Check sheet for the drawn part. Datum: minimum x, y, z corner. Units: mm. A direction names the side the tool comes from. Give positions to 0.01 mm unless a question says otherwise; leave off trailing zeros. Loops run counter-clockwise (first coordinate to the right, second up) from the corner with the lowest first, then second, coordinate; pieces in that order, holes last.
1. Cross-section at D-D, the plane x = 67.5. Record the cut outline in (y, z), plus the area to 3 significant figures.
2. Go/stop test with flat-tipped pins: pin 1 Ø5 at (y, z) = (22.5, 73.4) entering from -X; pin 2 Ø4 at (x, z) = (67.5, 12.5) entering from +Y; pin 3 Ø1.5 at (x, y) = (76.5, 78.5) entering from +Z; pin 4 Ø2.5 at (x, y) = (6.6, 22.5) entering from +Z. Record where each tip stops, or that it passes through.
3. Material ranges on L1, parallel to Z at x = 67.5, y = 14; L2, parallel to Y at x = 78.8, z = 12.5; L3, parallel to Y at x = 78, z = 12, recorded low to high.
4. Tool access check on the marked faces 1, 2 and 3. Record the directions out of +Z, -Z, +X, -X, +Y, -Y that give a thin tool (end or side, any length) a straight path to the whole face; none if there is none.
5. Cross-section at B-B, the plane x = 6.6. Record the cut outline in (y, z), plus the area to 3 significant figures.
6. Cross-section at A-A, the plane y = 22.5. Record the cut outline in (x, z).
7. Cross-section at C-C, the plane z = 73.4. Record the cut outline in (x, y).
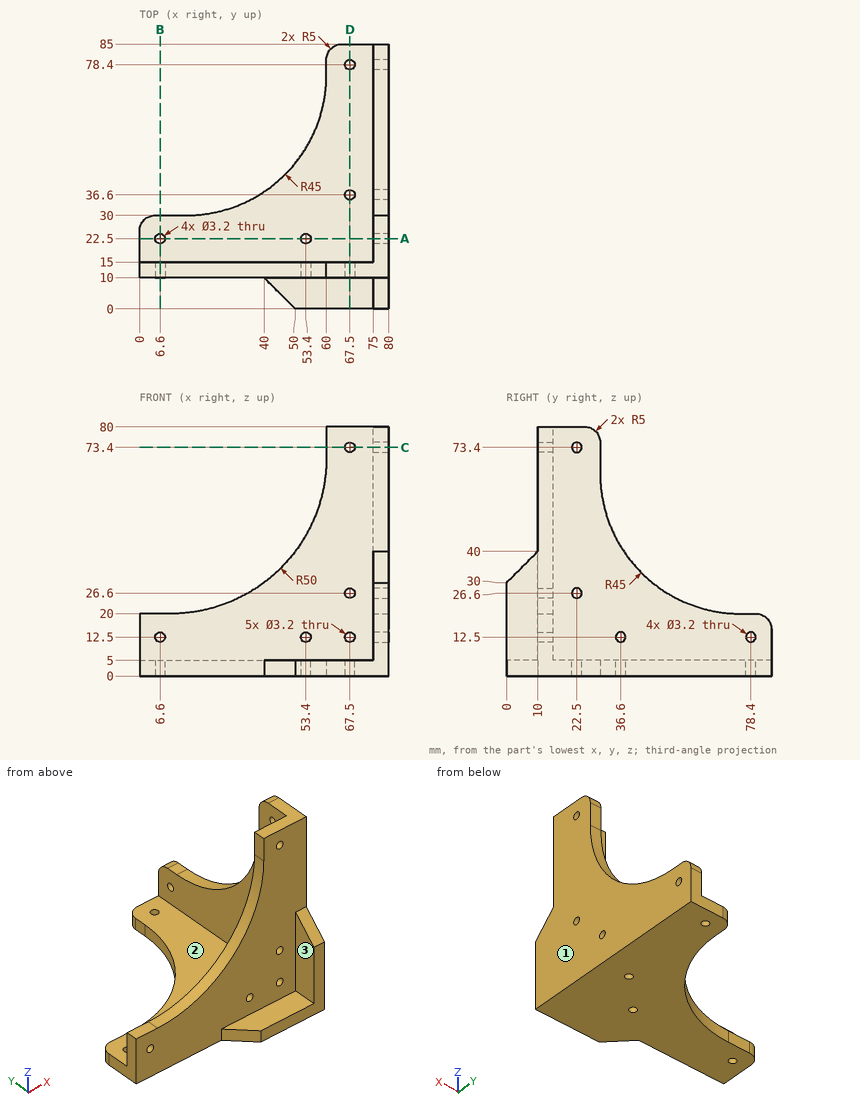
Result:
1. outline: (0, 0) - (35, 0) - (35, 5) - (15, 5) - (15, 10.9) - (10, 10.9) - (10, 5) - (0, 5) - close; (10, 14.1) - (15, 14.1) - (15, 25) - (10, 25) - close; (10, 28.2) - (15, 28.2) - (15, 71.8) - (10, 71.8) - close; (10, 75) - (15, 75) - (15, 80) - (10, 80) - close; (38.2, 0) - (76.8, 0) - (76.8, 5) - (38.2, 5) - close; (80, 0) - (85, 0) - (85, 5) - (80, 5) - close
1. area: 720 mm2
2. pin 1: stops at x = 75
2. pin 2: stops at y = 15
2. pin 3: stops at z = 20
2. pin 4: passes through
3. L1: z = 0 to 10.9, 14.1 to 25, 28.2 to 71.8, 75 to 80
3. L2: y = 0 to 35, 38.2 to 76.8, 80 to 85
3. L3: y = 0 to 35.08, 38.12 to 76.88, 79.92 to 85
4. face 1: +Z, -Z, +X, +Y, -Y
4. face 2: +Z, -X, +Y
4. face 3: +Z, -X, -Y
5. outline: (10, 0) - (20.9, 0) - (20.9, 5) - (15, 5) - (15, 10.9) - (10, 10.9) - close; (10, 14.1) - (15, 14.1) - (15, 20) - (10, 20) - close; (24.1, 0) - (30, 0) - (30, 5) - (24.1, 5) - close
5. area: 143 mm2
6. outline: (0, 0) - (5, 0) - (5, 5) - (0, 5) - close; (8.2, 0) - (51.8, 0) - (51.8, 5) - (8.2, 5) - close; (55, 0) - (80, 0) - (80, 25) - (75, 25) - (75, 5) - (55, 5) - close; (75, 28.2) - (80, 28.2) - (80, 71.8) - (75, 71.8) - close; (75, 75) - (80, 75) - (80, 80) - (75, 80) - close
7. outline: (60, 10) - (65.9, 10) - (65.9, 15) - (60, 15) - close; (69.1, 10) - (80, 10) - (80, 20.9) - (75, 20.9) - (75, 15) - (69.1, 15) - close; (75, 24.1) - (80, 24.1) - (80, 30) - (75, 30) - close
